```python
from build123d import *

# Parameters (mm, degrees)
F0_W     = 20.5
F0_H     = 47
F1_DEPTH = 22
F0_H_2   = 13
F2_DEPTH = 7
F3_DEPTH = 71
F4_W     = 17.699432
F4_H     = 29.777118
F5_DEPTH = 20
F6_R     = 5
F7_DEPTH = 10
F8_R     = 2.998853
F9_DEPTH = 10


with BuildPart() as f1:
    # F0 (on Top) → F1 (new body)
    with BuildSketch(Plane.XY):
        Rectangle(F0_W, F0_H)
    extrude(amount=-F1_DEPTH)

    # F0 (on Top) → F2 (join)
    with BuildSketch(Plane.XY):
        with Locations((0, -30)):
            Rectangle(F0_W, F0_H_2)
        with BuildLine():
            ThreePointArc((-6.25, -31.5), (-8.75, -29), (-6.25, -26.5))
            Line((-6.25, -26.5), (6.25, -26.5))
            ThreePointArc((6.25, -26.5), (8.017767, -27.232233), (8.75, -29))
            ThreePointArc((8.75, -29), (8.017767, -30.767767), (6.25, -31.5))
            Line((6.25, -31.5), (-6.25, -31.5))
        make_face(mode=Mode.SUBTRACT)
        with Locations((0, 30)):
            Rectangle(F0_W, F0_H_2)
        with BuildLine():
            ThreePointArc((6.25, 31.5), (8.017767, 30.767767), (8.75, 29))
            ThreePointArc((8.75, 29), (8.017767, 27.232233), (6.25, 26.5))
            Line((6.25, 26.5), (-6.25, 26.5))
            ThreePointArc((-6.25, 26.5), (-8.75, 29), (-6.25, 31.5))
            Line((-6.25, 31.5), (6.25, 31.5))
        make_face(mode=Mode.SUBTRACT)
    extrude(amount=-F2_DEPTH)

    # F0 (on Top) → F3 (join)
    with BuildSketch(Plane.XY):
        Polygon((-10.25, 36.5), (-11.75, 36.5), (-11.75, -36.5), (-10.25, -36.5), (-10.25, -23.5), (-10.25, 23.5), align=None)
        Polygon((11.75, 36.5), (10.25, 36.5), (10.25, 23.5), (10.25, -23.5), (10.25, -36.5), (11.75, -36.5), align=None)
    extrude(amount=-F3_DEPTH)

    # F4 (on face) → F5 (join)
    with BuildSketch(Plane(origin=(0, 0, -22), x_dir=(1, 0, 0), z_dir=(0, 0, -1))):
        Rectangle(F4_W, F4_H)
    extrude(amount=F5_DEPTH)

    # F6 (on face) → F7 (cut)
    with BuildSketch(Plane.XZ.offset(14.888559)):
        with Locations((0, -32)):
            Circle(F6_R)
    extrude(amount=-F7_DEPTH, mode=Mode.SUBTRACT)

    # F8 (on face) → F9 (cut)
    with BuildSketch(Plane(origin=(0, 14.888559, 0), x_dir=(-1, 0, 0), z_dir=(0, 1, 0))):
        with Locations((4.424858, -27)):
            Circle(F8_R)
        with Locations((4.424858, -37)):
            Circle(F8_R)
        with Locations((-4.424858, -37)):
            Circle(F8_R)
        with Locations((-4.424858, -27)):
            Circle(F8_R)
    extrude(amount=-F9_DEPTH, mode=Mode.SUBTRACT)


solid = f1.part
```
Model file for the job. Use its own axes, mm. A direction names the side the tool comes from. Coordinates: 2 decimals unless noted, no trailing zeros. Loops run counter-clockwise (first coordinate to the right, second up) from the corner with the lowest first, then second, coordinate; pieces in that order, holes last. Notation, with made-up numbers: (-37, 87.5) - (4, 87.5) arc R6 cw to (4, 97.5) - close; hole circle Ø8 at (61.5, -39.5). An arc over 180 degrees is marked (long way). Answer as a JSON object with one key per item and string values. Group by question number.
(1) Cut at D-D (y = 11). Give the cut face in (x, z).
(2) Tool access for faces 4 (the face through (0, 32, -7)), 5 (the face through (0, 0, -42)), 6 (the face through (-1.08, -9.96, -36.88)): list every direction of +Z, -Z, +X, -X, +Y, -Y with a clear straight run to the whole face (end or side of a thin tool).
(3) Flat gauge pins, fed straight in: pin 1 (5 mm diameter, centred on x = 4, z = -38.5, fed in from +Y); pin 2 (6 mm diameter, centred on x = -6, y = 26, fed in from -Z); pin 3 (3.5 mm diameter, centred on x = 4.42, z = -27, fed in from +Y); pin 4 (3 mm diameter, centred on x = -8, z = -50, fed in from +Y). Where does each tip first touch, or does it go through?
(4) Cut at C-C (y = -12). Give the cut face in (x, z), then the cut area to 3 significant figures.
(5) Two-plate mould, pull along Z, no slides. Class faces 1 (the face through (4, 4.889, -27)), 2 (the face through (-10.25, -1, -39)), 3 (the face through (0, -33, -7)): released by +Z, released by -Z, zero draft, split by the parting line, or undercut.
(6) Cut at A-A (z = -58.5). Give the cut face in (x, y), then the cut area to 3 significant figures.
(7) Cut at B-B (x = 0). Give the cut face in (y, z).
(8) Probe line 1 along X through (y, z) = (32, -43.5); line 2 along X through (y, z) = (12.5, -23); line 3 along Z through (x, y) = (0, -8.25). List the from-to ranges inside material, lowest first.
Geometry says:
{
 "1": {"outline": "(-11.75, -71) - (-10.25, -71) - (-10.25, -22) - (-8.85, -22) - (-8.85, -42) - (8.85, -42) - (8.85, -22) - (10.25, -22) - (10.25, -71) - (11.75, -71) - (11.75, 0) - (-11.75, 0) - close; hole circle Ø6 at (-4.42, -37); hole circle Ø6 at (-4.42, -27); hole circle Ø6 at (4.42, -37); hole circle Ø6 at (4.42, -27)"},
 "2": {"face 4": "-Z, +Y", "face 5": "-Z, +Y, -Y", "face 6": "-Y"},
 "3": {"pin 1": "stops at y = 14.89", "pin 2": "stops at z = -22", "pin 3": "stops at y = 4.89", "pin 4": "passes through"},
 "4": {"outline": "(-11.75, -71) - (-10.25, -71) - (-10.25, -22) - (-8.85, -22) - (-8.85, -42) - (8.85, -42) - (8.85, -22) - (10.25, -22) - (10.25, -71) - (11.75, -71) - (11.75, 0) - (-11.75, 0) - close; hole circle Ø10 at (0, -32)", "area": "939 mm^2"},
 "5": {"face 1": "undercut", "face 2": "zero draft", "face 3": "released by -Z"},
 "6": {"outline": "(-11.75, -36.5) - (-10.25, -36.5) - (-10.25, 36.5) - (-11.75, 36.5) - close; (10.25, -36.5) - (11.75, -36.5) - (11.75, 36.5) - (10.25, 36.5) - close", "area": "219 mm^2"},
 "7": {"outline": "(-36.5, -7) - (-31.5, -7) - (-31.5, 0) - (-36.5, 0) - close; (-26.5, -7) - (-23.5, -7) - (-23.5, -22) - (-14.89, -22) - (-14.89, -27) - (-4.89, -27) - (-4.89, -37) - (-14.89, -37) - (-14.89, -42) - (14.89, -42) - (14.89, -22) - (23.5, -22) - (23.5, -7) - (26.5, -7) - (26.5, 0) - (-26.5, 0) - close; (31.5, -7) - (36.5, -7) - (36.5, 0) - (31.5, 0) - close"},
 "8": {"line 1": "x = -11.75 to -10.25, 10.25 to 11.75", "line 2": "x = -11.75 to -10.25, -8.85 to 8.85, 10.25 to 11.75", "line 3": "z = -42 to -37, -27 to 0"}
}
